from build123d import *

# Parameters (mm, degrees)
F1_W     = 30
F1_H     = 30
F2_DEPTH = 5
F3_DEPTH = 15
F4_R     = 0.49999


# Not quite as in the source:
# - a fillet or chamfer is up to 0.001 mm smaller than in the source, because OpenCascade refuses the exact size


with BuildPart() as f2:
    # F1 (on Top) → F2 (new body)
    with BuildSketch(Plane.XY):
        Rectangle(F1_W, F1_H)
    extrude(amount=-F2_DEPTH)

    # F0 (on Front) → F3 (join, symmetric)
    with BuildSketch(Plane.XZ):
        with BuildLine():
            ThreePointArc((0, 0), (-10.4582503317, 5.6534680312), (-11.4564392374, 17.5))
            Line((-11.4564392374, 17.5), (-12.539936204, 17.5))
            ThreePointArc((-12.539936204, 17.5), (-13.257811636, 15.0456689932), (-13.5, 12.5))
            Line((-13.5, 12.5), (-13.5, 0))
            Line((-13.5, 0), (0, 0))
        make_face()
        with BuildLine():
            ThreePointArc((11.4564392374, 17.5), (10.4582503317, 5.6534680312), (0, 0))
            Line((0, 0), (13.5, 0))
            Line((13.5, 0), (13.5, 12.5))
            ThreePointArc((13.5, 12.5), (13.257811636, 15.0456689932), (12.539936204, 17.5))
            Line((12.539936204, 17.5), (11.4564392374, 17.5))
        make_face()
    extrude(amount=F3_DEPTH, both=True)

    # F4 (radius 0.5 in the source; OpenCascade refuses exactly that, so slightly less here)
    f4_edges = [f2.edges().sort_by_distance(p)[0] for p in [
        (-11.456439, 0, 17.5),
        (12.539936, 0, 17.5),
        (-12.539936, 0, 17.5),
        (11.456439, 0, 17.5),
    ]]
    fillet(f4_edges, radius=F4_R)


solid = f2.part
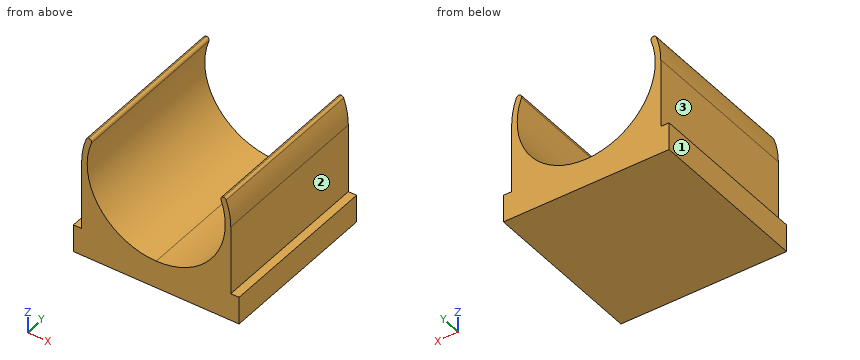
Source: CAD feature listing. Evaluate the final solid. Frame: model axes, mm. Face numbers are marked on the shaded views. A direction names the side the tool comes from. Round coordinates to 2 decimals unless told otherwise and drop trailing zeros. Loops run counter-clockwise (first coordinate to the right, second up) from the corner with the lowest first, then second, coordinate; pieces in that order, holes last.
Q1. Section D-D, the plane x = -2.5. Return loops of the section in (y, z), plus the area to 3 significant figures.
Q2. Section B-B, the plane z = 6. Return loops of the section in (x, y), plus the area to 3 significant figures.
Q3. First-contact query: P1, Ø1, axis at y = 6, z = 11, coming from the -X side; P2, Ø12, axis at x = -1, y = -4, coming from the +Z side; P3, Ø0.8, axis at x = 14.5, y = 4, coming from the +Z side. Flat tips, straight axial feed; report the tip coordinate or a pass-through.
Q4. Ray query, line 1 (X direction, y = -0.25, z = 12.75); line 2 (X direction, y = -6.5, z = 15.75); line 3 (Z direction, x = -9, y = 6.5). Return the intervals inside material, ascending.
Q5. Section A-A, the plane z = 12. Return loops of the section in (x, y), plus the area to 3 significant figures.
Q6. Access query for the marked faces 1, 2 and 3. Directions: +Z, -Z, +X, -X, +Y, -Y. A direction counts if a zero-diameter tool reaches every point of the face in a straight line with its end or side. Return the directions, or none.
Solutions:
1. outline: (-15, -5) - (15, -5) - (15, 0.25) - (-15, 0.25) - close
1. area: 158 mm2
2. outline: (-13.5, -15) - (-10.68, -15) - (-10.68, 15) - (-13.5, 15) - close; (10.68, -15) - (13.5, -15) - (13.5, 15) - (10.68, 15) - close
2. area: 169 mm2
3. P1: stops at x = -13.5
3. P2: stops at z = 2.14
3. P3: stops at z = 0
4. line 1: x = -13.5 to -12.5, 12.5 to 13.5
4. line 2: x = -13.1 to -12.07, 12.07 to 13.1
4. line 3: z = -5 to 3.83
5. outline: (-13.5, -15) - (-12.49, -15) - (-12.49, 15) - (-13.5, 15) - close; (12.49, -15) - (13.5, -15) - (13.5, 15) - (12.49, 15) - close
5. area: 60.6 mm2
6. face 1: +Z, -Z, -X, +Y, -Y
6. face 2: +Z, +X, +Y, -Y
6. face 3: +Z, -X, +Y, -Y
